from build123d import *

# Parameters (mm, degrees)
SKETCH_1_W          = 56
SKETCH_1_H          = 25
EXTRUDE_1_DEPTH     = 2
SKETCH_2_R          = 1.45
EXTRUDE_2_DEPTH     = 2
SKETCH_3_R          = 1.55
SKETCH_3_R_2        = 4.1
CUT_EXTRUDE_1_DEPTH = 2
FILLET_1_R          = 2
EXTRUDE_START       = 2.5
SKETCH_4_W          = 13
SKETCH_4_H          = 25
SKETCH_4_R          = 1.55
EXTRUDE_3_DEPTH     = 2.5
CHAMFER_1_SIZE      = 2


with BuildPart() as part:
    # Sketch 1 → Extrude 1 (new body)
    with BuildSketch(Plane.XY):
        Rectangle(SKETCH_1_W, SKETCH_1_H)
    extrude(amount=EXTRUDE_1_DEPTH)

    # Sketch 2 → Extrude 2 (add)
    with BuildSketch(Plane(origin=(28, 0, 0), x_dir=(0, 0, -1), z_dir=(1, 0, 0))):
        with BuildLine():
            Line((16, 12.5), (0, 12.5))
            Line((0, 12.5), (0, -12.5))
            Line((0, -12.5), (16, -12.5))
            ThreePointArc((16, -12.5), (21.8630197, -11.039701083), (26.356157589, -7))
            ThreePointArc((26.356157589, -7), (27.31423641, -5.313949046), (28, -3.5))
            ThreePointArc((28, -3.5), (28.374368671, -1.767766953), (28.5, 0))
            ThreePointArc((28.5, 0), (24.838834765, 8.838834765), (16, 12.5))
        make_face()
        with Locations((9, 0)):
            Circle(SKETCH_2_R, mode=Mode.SUBTRACT)
        with Locations((16, -7)):
            Circle(SKETCH_2_R, mode=Mode.SUBTRACT)
        with BuildLine():
            ThreePointArc((16, 4.1), (18.899137803, 2.899137803), (20.1, 0))
            ThreePointArc((20.1, 0), (13.100862197, -2.899137803), (16, 4.1))
        make_face(mode=Mode.SUBTRACT)
        with BuildLine():
            ThreePointArc((24.45, 0), (23, -1.45), (21.55, 0))
            ThreePointArc((21.55, 0), (23, 1.45), (24.45, 0))
        make_face(mode=Mode.SUBTRACT)
        with BuildLine():
            ThreePointArc((17.45, 7), (17.025304833, 5.974695167), (16, 5.55))
            ThreePointArc((16, 5.55), (14.974695167, 5.974695167), (14.55, 7))
            ThreePointArc((14.55, 7), (14.974695167, 8.025304833), (16, 8.45))
            ThreePointArc((16, 8.45), (17.025304833, 8.025304833), (17.45, 7))
        make_face(mode=Mode.SUBTRACT)
    extrude_2 = extrude(amount=-EXTRUDE_2_DEPTH)

    # Mirror 2: Extrude 2 across plane
    add(extrude_2.mirror(Plane.ZY))

    # Sketch 3 → Cut-Extrude 1 (cut)
    with BuildSketch(Plane.XY.offset(2)):
        with Locations((-20, 0)):
            Circle(SKETCH_3_R)
        with Locations((-6.5, 0)):
            Circle(SKETCH_3_R)
        with Locations((6.5, 0)):
            Circle(SKETCH_3_R)
        with Locations((0, -6.5)):
            Circle(SKETCH_3_R)
        Circle(SKETCH_3_R_2)
        with Locations((0, 6.5)):
            Circle(SKETCH_3_R)
        with Locations((20, 0)):
            Circle(SKETCH_3_R)
    extrude(amount=-CUT_EXTRUDE_1_DEPTH, mode=Mode.SUBTRACT)

    # Fillet 1
    fillet_1_edges = [part.edges().sort_by_distance(p)[0] for p in [
        (26, 0, 0),
        (-26, 0, 0),
    ]]
    fillet(fillet_1_edges, radius=FILLET_1_R)

    # Sketch 4 → Extrude 3 (add)
    # profile 1 of 2: a face of its own
    with BuildSketch(Plane.XY.offset(2).offset(EXTRUDE_START)):
        with Locations((-21.5, 0)):
            Rectangle(SKETCH_4_W, SKETCH_4_H)
        with Locations((-20, 0)):
            Circle(SKETCH_4_R, mode=Mode.SUBTRACT)
    # profile 2 of 2: a face of its own
    with BuildSketch(Plane.XY.offset(2).offset(EXTRUDE_START)):
        with Locations((21.5, 0)):
            Rectangle(SKETCH_4_W, SKETCH_4_H)
        with Locations((20, 0)):
            Circle(SKETCH_4_R, mode=Mode.SUBTRACT)
    extrude(amount=-EXTRUDE_3_DEPTH)

    # Chamfer 1
    chamfer_1_edges = [part.edges().sort_by_distance(p)[0] for p in [
        (-28, 0, 4.5),
        (28, 0, 4.5),
    ]]
    chamfer(chamfer_1_edges, length=CHAMFER_1_SIZE)


solid = part.part
Here's how the part is built. I have some questions about the finished solid (model axes, mm). A direction names the side the tool comes from. Coordinates: 2 decimals unless noted, no trailing zeros. Loops run counter-clockwise (first coordinate to the right, second up) from the corner with the lowest first, then second, coordinate; pieces in that order, holes last.
1. I need wall thicknesses on L1, parallel to Y at x = 27.35, z = -16; L2, parallel to Y at x = 6.5, z = 0.65; L3, parallel to X at y = -3.75, z = -10.5. Which ranges of each line are inside material? Lowest first, please.
2. Imagine slicing it at B-B, the plane x = 0.5. Please give me the cut outline in (y, z).
3. For P1, Ø2, axis at x = -3.5, y = 5.5, coming from the +Z side; P2, Ø3, axis at y = -3.5, z = 3.5, coming from the +X side; P3, Ø4, axis at x = -1.5, y = 9.5, coming from the -Z side, each with a flat end and sliding along its axis, tell me the tip position at first contact or that it passes through.
4. If we mould it in two halves opening along Z, with no side actions, what happens to faces 1 (the flat face through (28, 3, -12.8)), 2 (the cylindrical face through (27.014, -7.555, -17.339)), 3 (the flat face through (-22, 0, 4.5))? For each: pulls with the +Z half, pulls with the -Z half, needs draft (parallel to the pull), parting line crosses it, or undercut.
5. Imagine slicing it at D-D, the plane x = -10. Please give me the cut outline in (y, z), and give its area (3 significant figures).
6. Imagine slicing it at C-C, the plane z = -13.5. Please give me the cut outline in (x, y), and give its area (3 significant figures).
7. For faces 4 (the flat face through (26, 3, -12)), 5 (the flat face through (-4, 3, 2)), 6 (the cylindrical face through (4.95, 0.07, 1.01)), which set-ups out of +Z, -Z, +X, -X, +Y, -Y let a thin tool reach every point of the face, with its end or its side?
8. Imagine slicing it at A-A, the plane x = -20. Please give me the cut outline in (y, z).
Taken from the geometry:
1. L1: y = -12.5 to -8.45, -5.55 to -4.1, 4.1 to 5.55, 8.45 to 12.5
1. L2: y = -12.5 to -1.55, 1.55 to 12.5
1. L3: x = -28 to -26, 26 to 28
2. outline: (-12.5, 0) - (-7.97, 0) - (-7.97, 2) - (-12.5, 2) - close; (-5.03, 0) - (-4.07, 0) - (-4.07, 2) - (-5.03, 2) - close; (4.07, 0) - (5.03, 0) - (5.03, 2) - (4.07, 2) - close; (7.97, 0) - (12.5, 0) - (12.5, 2) - (7.97, 2) - close
3. P1: stops at z = 2
3. P2: stops at x = 28
3. P3: stops at z = 0
4. face 1: needs draft
4. face 2: undercut
4. face 3: pulls with the +Z half
5. outline: (-12.5, 0) - (12.5, 0) - (12.5, 2) - (-12.5, 2) - close
5. area: 50.0 mm2
6. outline: (-28, -12.5) - (-26, -12.5) - (-26, -3.25) - (-28, -3.25) - close; (-28, 3.25) - (-26, 3.25) - (-26, 12.5) - (-28, 12.5) - close; (26, -12.5) - (28, -12.5) - (28, -3.25) - (26, -3.25) - close; (26, 3.25) - (28, 3.25) - (28, 12.5) - (26, 12.5) - close
6. area: 74.0 mm2
7. face 4: -Z, +Y, -Y
7. face 5: +Z, +Y, -Y
7. face 6: +Z, -Z
8. outline: (-12.5, 0) - (-1.55, 0) - (-1.55, 4.5) - (-12.5, 4.5) - close; (1.55, 0) - (12.5, 0) - (12.5, 4.5) - (1.55, 4.5) - close
